Read the model definition and answer for the solid it produces. Units are mm, in the model's axes. A direction names the side the tool comes from. Round coordinates to 2 decimals unless told otherwise and drop trailing zeros. Write each loop counter-clockwise with the first axis right and the second up, starting at its lowest first coordinate (ties: lowest second). Pieces come first, ordered by that corner, then holes. Notation, with made-up numbers: (-37.5, 1.25) -> (1.5, 1.25) arc R14 cw to (1.5, 21.25) -> close; hole circle Ø2 at (-9, -4). An arc over 180 degrees is marked (long way). Return JSON: item names as keys, results as strings.
Autodesk Inventor part; units mm, degrees
ref_plane "YZ Plane" through (0, 0, 0) normal (1, 0, 0) x (0, 1, 0)
ref_plane "XZ Plane" through (0, 0, 0) normal (0, 1, 0) x (-1, 0, 0)
ref_plane "XY Plane" through (0, 0, 0) normal (0, 0, 1) x (1, 0, 0)
sketch "Sketch1" plane through (0, 0, 0) normal (0, 0, 1) x (1, 0, 0)
  circle A0 centre (0, 0) radius 5
  dimension "d0" = 10
extrude "Extrusion1" add sketch "Sketch1" along normal blind 5
sketch "Sketch2" plane through (0, 0, 5) normal (0, 0, 1) x (1, 0, 0)
  line L0 (-1.5, -5) -> (1.5, -5)
  line L1 (1.5, -5) -> (1.5, 5)
  line L2 (1.5, 5) -> (-1.5, 5)
  line L3 (-1.5, 5) -> (-1.5, -5)
  line L4 (-1.5, -5) -> (1.5, 5) construction
  line L5 (1.5, -5) -> (-1.5, 5) construction
  circle A0 centre (0, 0) radius 5
  dimension "d3" = 3
  dimension "d4" = 10
extrude "Extrusion2" add sketch "Sketch2" along normal blind 10 contours L3 A0 L0 | A0 L1 L0 | A0 L3 L1 | L3 L2 A0 | A0 L2 L1
sketch "Sketch3" plane through (1.5, -4.7697, 5) normal (1, 0, 0) x (0, 0, -1)
  line L0 (0, -0.2303) -> (-10, -0.2303)
  line L1 (-10, 9.7697) -> (0, -0.2303)
  line L2 (0, -0.2303) -> (0, 9.7697)
  line L3 (-10, 9.7697) -> (-10, -0.2303)
  line L4 (0, 9.7697) -> (-10, -0.2303)
  circle A0 centre (-5, 4.7697) radius 1.5
  point P0 (5, 4.7697)
  dimension "d7" = 3
extrude "Extrusion3" cut sketch "Sketch3" against normal through all contours A0 L4 L1 | L1 L4 A0 | A0 L1 L4 | L1 A0 L4
sketch "Sketch4" plane through (1.5, -4.7697, 5) normal (1, 0, 0) x (0, 0, -1)
  circle A0 centre (-5, 4.7697) radius 1.5
  circle A1 centre (-5, 4.7697) radius 5
  line L0 (-5, 4.7697) -> (-5, 9.7697)
  line L1 (-5, 4.7697) -> (-5, -0.2303)
  line L2 (0, -0.2303) -> (-10, -0.2303)
  line L3 (-10, -0.2303) -> (-10, 9.7697)
  line L4 (0, 9.7697) -> (-10, 9.7697)
  point P0 (5, 4.7697)
  point P1 (-10, 4.7697)
extrude "Extrusion4" cut sketch "Sketch4" against normal through all contours A1 L3 L4 | L2 L3 A1
properties part number "pm connector"
Item 1: Straight lines are drawn through the part: L1, parallel to Y at x = -0.35, z = 10; L2, parallel to Z at x = 0.55, y = 0; L3, parallel to X at y = 1.75, z = 13. For each, find the intervals that lie inside material, in ascending order. Write a range as [from, to].
Worked answers:
{"L1": "y = [-5, -1.5], [1.5, 5]", "L2": "z = [0, 8.5], [11.5, 15]", "L3": "x = [-1.5, 1.5]"}
Item 2: Section A-A (y = 0) is taken. Give the vertices of the cut face in (x, z), then the cut area to 3 significant figures.
Worked answers:
{"outline": "(-5, 0) -> (5, 0) -> (5, 5) -> (1.5, 5) -> (1.5, 8.5) -> (-1.5, 8.5) -> (-1.5, 5) -> (-5, 5) -> close; (-1.5, 11.5) -> (1.5, 11.5) -> (1.5, 15) -> (-1.5, 15) -> close", "area": "71.0 mm2"}
Item 3: Section C-C (z = 10.5) is taken. Give the vertices of the cut face in (x, y), then the cut area to 3 significant figures.
Worked answers:
{"outline": "(-1.5, -4.97) -> (1.5, -4.97) -> (1.5, -1.41) -> (-1.5, -1.41) -> close; (-1.5, 1.41) -> (1.5, 1.41) -> (1.5, 4.97) -> (-1.5, 4.97) -> close", "area": "21.4 mm2"}
Item 4: Flat-ended cylindrical pins translate along their axes: pin 1 (2.5 mm diameter, centred on y = 0, z = 10, fed in from -X); pin 2 (1.5 mm diameter, centred on x = -3, z = 4.5, fed in from -Y); pin 3 (3 mm diameter, centred on y = 4, z = 2.5, fed in from -X); pin 4 (1.8 mm diameter, centred on x = -3.5, y = 0.5, fed in from +Z). Find the tip coordinate at first contact, or state that the pin passes through.
Worked answers:
{"pin 1": "passes through", "pin 2": "stops at y = -4.47", "pin 3": "stops at x = -4.33", "pin 4": "stops at z = 5"}
Item 5: For a pull along Z with two mould halves and no side action, classify faces 4 (the flat face through (-1.5, 1.2, 8.8)), 5 (the flat face through (0, 0, 0)), 6 (the cylindrical face through (0.02, 0.07, 11.5)), 7 (the flat face through (3, 0, 5)) as released by +Z, released by -Z, zero draft, split by the parting line, or undercut.
Worked answers:
{"face 4": "zero draft", "face 5": "released by -Z", "face 6": "undercut", "face 7": "released by +Z"}
Item 6: Section D-D (y = 3.5) is taken. Give the vertices of the cut face in (x, z), then the cut area to 3 significant figures.
Worked answers:
{"outline": "(-3.57, 0) -> (3.57, 0) -> (3.57, 5) -> (1.5, 5) -> (1.5, 13.57) -> (-1.5, 13.57) -> (-1.5, 5) -> (-3.57, 5) -> close", "area": "61.4 mm2"}
Item 7: A tool of negligible diameter and unlimited length cuts with its end or side. For faces 1 (the flat face through (1.5, -1.2, 8.8)), 2 (the flat face through (-3, 0, 5)), 3 (the cylindrical face through (-1.08, 4.88, 2.46)), from which of +Z, -Z, +X, -X, +Y, -Y can it reach the whole face along a straight path? Write none if from no direction.
Worked answers:
{"face 1": "+Z, +X, +Y, -Y", "face 2": "+Z, -X, +Y, -Y", "face 3": "-Z"}
